Job drawing, mm, ordinate dimensions from the low corner. One solid piece. Coordinates: 2 decimals unless noted, no trailing zeros. Write each loop counter-clockwise with the first axis right and the second up, starting at its lowest first coordinate (ties: lowest second). Pieces come first, ordered by that corner, then holes. Notation, with made-up numbers: (15, 4.5) -> (30, 4.5) arc R20 cw to (30, 8.5) -> close; hole circle Ø2 at (23.5, 60). An arc over 180 degrees is marked (long way). One line per question, with ' | ' between items. Start each with the question number.
Item 1: Pin check, flat tips, straight feed: pin 1 (8 mm diameter, centred on x = 230.5, z = 69, fed in from -Y) (3 decimals); pin 2 (3 mm diameter, centred on x = 133.5, z = 63, fed in from -Y); pin 3 (10 mm diameter, centred on x = 187.5, z = 89.5, fed in from +Y). Stop position of each tip, or through.
Item 2: Saw through at B-B (z = 86). List the corners of the cut face in (x, y).
Item 3: Probe probe 1 along Y at (x, z) = (133, 53); probe 2 along Z at (x, y) = (174.5, 52.5); probe 3 along Z at (x, y) = (246.5, 46.5). List the from-to ranges inside material, lowest first. Write a range as [from, to].
Item 4: Saw through at A-A (x = 269). List the corners of the cut face in (y, z), and give its area (3 significant figures).
Item 5: Saw through at C-C (y = 32). List the corners of the cut face in (x, z).
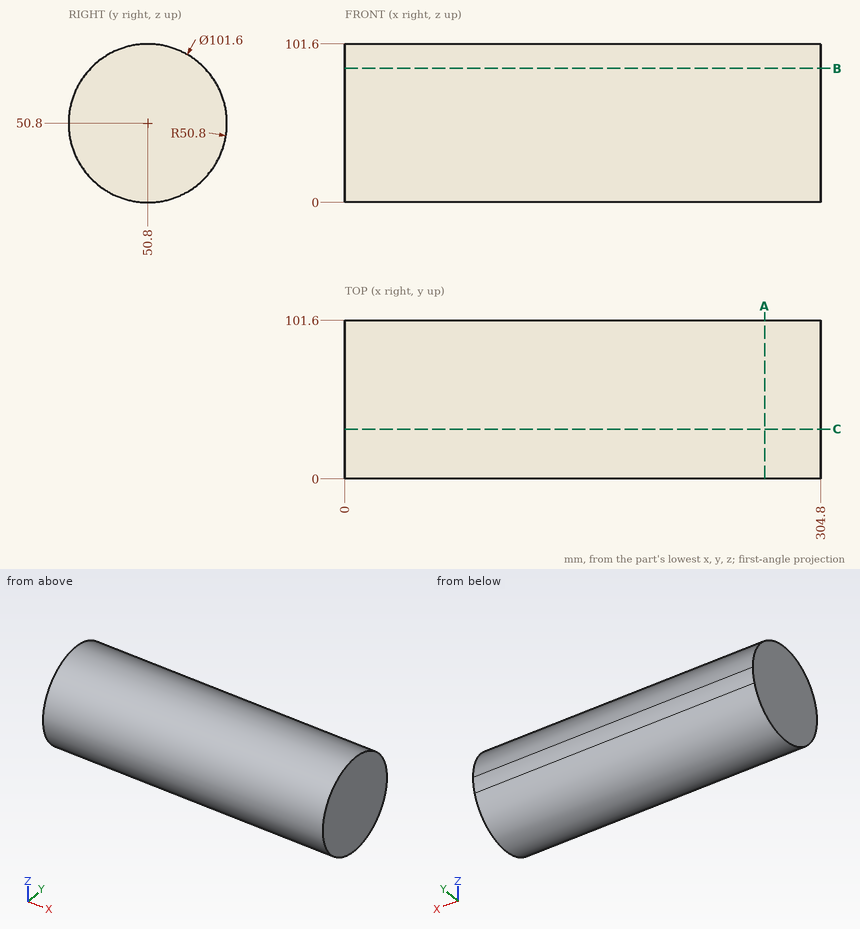
From the geometry:
1) pin 1: y = 2.025 | pin 2: y = 1.14 | pin 3: y = 88.81
2) outline: (0, 14.17) -> (304.8, 14.17) -> (304.8, 87.43) -> (0, 87.43) -> close
3) probe 1: [0.05, 101.55] | probe 2: [0.03, 101.57] | probe 3: [0.18, 101.42]
4) outline: circle Ø101.6 at (50.8, 50.8) | area: 8,110 mm2
5) outline: (0, 3.61) -> (304.8, 3.61) -> (304.8, 97.99) -> (0, 97.99) -> close
